Read the model definition and answer for the solid it produces. Units are mm, in the model's axes. Round coordinates to 2 decimals unless told otherwise and drop trailing zeros. Order: outer loops, then holes, each group sorted by start corner. A loop starts at its lowest first (then second) coordinate and runs counter-clockwise, first axis right, second up. Notation, with made-up numbers: M -24.75,53 L -8.75,53 A24 ccw -8.75,77 Z; hole C 87.5,54 d5. An arc over 180 degrees is marked long. Answer as CSV lines item,"result".
```python
from build123d import *

# Parameters (mm, degrees)
SKETCH1_W               = 180
SKETCH1_H               = 180
BOSS_EXTRUDE1_DEPTH     = 3
CUT_EXTRUDE1_DEPTH      = 128.314571044
CUT_EXTRUDE1_DEPTH_BACK = 128.314571044
SKETCH2_R               = 4
SKETCH2_R_2             = 1.5


with BuildPart() as part:
    # Sketch1 → Boss-Extrude1 (new body)
    with BuildSketch(Plane(origin=(0, 0, 0), x_dir=(1, 0, 0), z_dir=(0, 1, 0))):
        Rectangle(SKETCH1_W, SKETCH1_H)
    extrude(amount=BOSS_EXTRUDE1_DEPTH)

    # Sketch2 → Cut-Extrude1 (cut, two sides: drawn at the far end of the back side and taken through both)
    with BuildSketch(Plane(origin=(0, 3, 0), x_dir=(1, 0, 0), z_dir=(0, 1, 0)).offset(-CUT_EXTRUDE1_DEPTH_BACK)):
        with Locations(Location((0, 0, 0), (0, 0, 270))):
            Circle(SKETCH2_R)
        with Locations(Location((-16, 16, 0), (0, 0, 270))):
            Circle(SKETCH2_R_2)
        with Locations(Location((16, 16, 0), (0, 0, 270))):
            Circle(SKETCH2_R_2)
        with Locations(Location((16, -16, 0), (0, 0, 270))):
            Circle(SKETCH2_R_2)
        with Locations(Location((-16, -16, 0), (0, 0, 270))):
            Circle(SKETCH2_R_2)
    extrude(amount=CUT_EXTRUDE1_DEPTH + CUT_EXTRUDE1_DEPTH_BACK, mode=Mode.SUBTRACT)


solid = part.part
```
Item 1: Find the intervals of material crossed by probe 1 along Z at (x, y) = (16, 0.75); probe 2 along X at (y, z) = (1.85, 0), in increasing order. Write a range as [from, to].
Ans:
probe 1,"[-90, -17.5], [-14.5, 14.5], [17.5, 90]"
probe 2,"[-90, -4], [4, 90]"
Item 2: Determine the mould class of faces 1 (the face through (-3.905, 1.479, -0.867)), 2 (the face through (-1, 3, -21)) for opening direction X: +X half, -X half, draft (parallel to the pull), parting line (faces both ways), or undercut.
Ans:
face 1,"undercut"
face 2,"draft"
Item 3: A cutting plane is placed at B-B, the plane z = 0. Determine the outline of the cut face in (x, y), and give its area (3 significant figures).
Ans:
outline,"M -90,0 L -4,0 L -4,3 L -90,3 Z; M 4,0 L 90,0 L 90,3 L 4,3 Z"
area,"516 mm2"
Item 4: A cutting plane is placed at A-A, the plane x = 0. Determine the outline of the cut face in (y, z), and give its area (3 significant figures).
Ans:
outline,"M 0,-90 L 3,-90 L 3,-4 L 0,-4 Z; M 0,4 L 3,4 L 3,90 L 0,90 Z"
area,"516 mm2"
